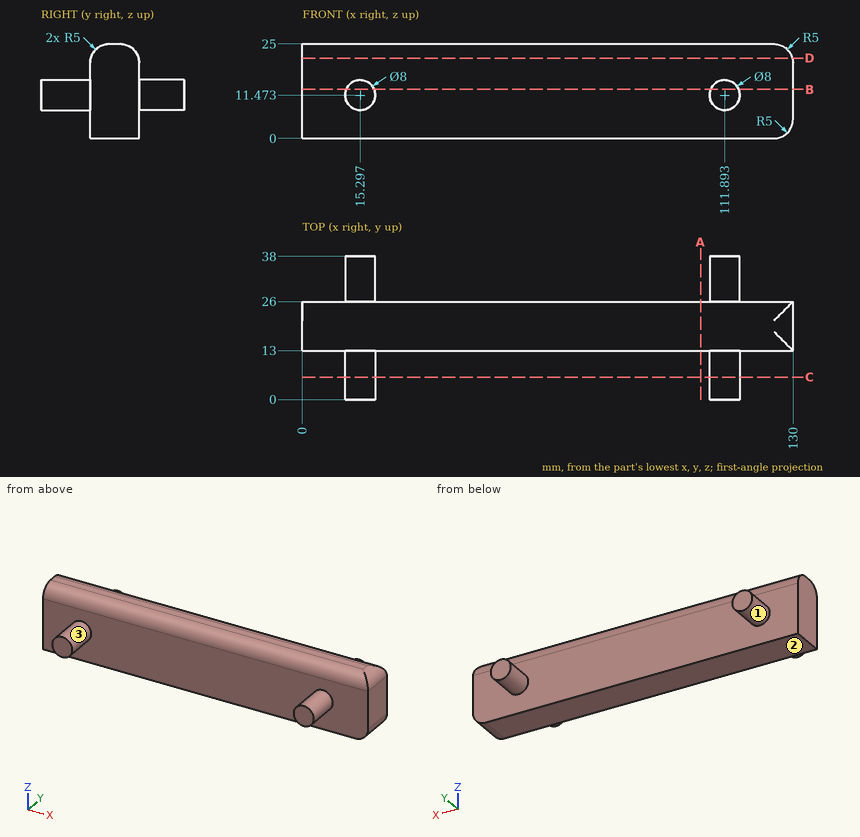
Design review of the part shown in the three views and the two pictorial views. Dimensions are in mm from the part's minimum x, y and z. A direction names the side the tool comes from. Round coordinates to 2 decimals unless told otherwise and drop trailing zeros. Loops run counter-clockwise (first coordinate to the right, second up) from the corner with the lowest first, then second, coordinate; pieces in that order, holes last. Notation, with made-up numbers: (-5, 11.5) -> (46, 11.5) arc R8 cw to (46, 16.5) -> close; hole circle Ø9 at (-27, 74). An arc over 180 degrees is marked (long way). Answer as a JSON object with one key per item and string values. Group by question number.
1) For line 1 (X direction, y = 4.5, z = 11) (1 decimal); line 2 (Z direction, x = 116.5, y = 21.5) (1 decimal); line 3 (Y direction, x = 10, z = 20), list the stretches that pass through material, from the lowest coordinate up. Write a range as [from, to].
2) For pin 1 Ø2 at (x, z) = (65.5, 6) entering from +Y; pin 2 Ø6 at (x, z) = (84.5, 4.5) entering from -Y, all flat-tipped, find the tip position at first contact; note any pin that passes through.
3) We need section A-A on x = 105.5. Write out the cut boundary in (y, z), then the cut area to 3 significant figures.
4) For the marked faces 1, 2 and 3, list the 3-axis set-ups (+Z, -Z, +X, -X, +Y, -Y) from which the entire face can be reached by the end or side of a thin tool; tool diameter is ignored.
5) We need section B-B on z = 13. Write out the cut boundary in (x, y), then the cut area to 3 significant figures.
6) We need section C-C on y = 6. Write out the cut boundary in (x, z).
7) We need section D-D on z = 21.25. Write out the cut boundary in (x, y).
Result set:
{
 "1": {"line 1": "[11.3, 19.3], [107.9, 115.9]", "line 2": "[0, 25]", "line 3": "[13, 26]"},
 "2": {"pin 1": "y = 26", "pin 2": "y = 13"},
 "3": {"outline": "(13, 0) -> (26, 0) -> (26, 20) arc R5 ccw to (21, 25) -> (18, 25) arc R5 ccw to (13, 20) -> close", "area": "314 mm²"},
 "4": {"face 1": "+Y", "face 2": "-Z, +X, -X, +Y, -Y", "face 3": "-Y"},
 "5": {"outline": "(0, 13) -> (11.6, 13) -> (11.6, 0) -> (18.99, 0) -> (18.99, 13) -> (108.2, 13) -> (108.2, 0) -> (115.59, 0) -> (115.59, 13) -> (130, 13) -> (130, 26) -> (115.59, 26) -> (115.59, 38) -> (108.2, 38) -> (108.2, 26) -> (18.99, 26) -> (18.99, 38) -> (11.6, 38) -> (11.6, 26) -> (0, 26) -> close", "area": "2,060 mm²"},
 "6": {"outline": "circle Ø8 at (15.3, 11.47); circle Ø8 at (111.89, 11.47)"},
 "7": {"outline": "(0, 13.16) -> (129.84, 13.16) -> (129.84, 25.84) -> (0, 25.84) -> close"}
}
